```python
from build123d import *

# Parameters (mm, degrees)
SKETCH1_W           = 288.2
SKETCH1_H           = 140
EXTRUDE_5_DEPTH     = 5
SKETCH2_W           = 10
SKETCH2_H           = 60
BOSS_EXTRUDE2_DEPTH = 5
SKETCH3_W           = 27
SKETCH3_H           = 4
SKETCH3_W_2         = 3
SKETCH3_H_2         = 7
CUT_EXTRUDE1_DEPTH  = 5
SKETCH4_R           = 8
CUT_EXTRUDE2_DEPTH  = 5
SKETCH5_R           = 2
CUT_EXTRUDE3_DEPTH  = 5
SKETCH6_W           = 50
SKETCH6_H           = 50
BOSS_EXTRUDE3_DEPTH = 5
LPATTERN1_COUNT     = 2
LPATTERN1_PITCH     = 105
FILLET1_R           = 10
FILLET2_R           = 10


with BuildPart() as part:
    # Sketch1 → Extrude 5 (new body)
    with BuildSketch(Plane(origin=(0, 0, 0), x_dir=(1, 0, 0), z_dir=(0, 1, 0))):
        Rectangle(SKETCH1_W, SKETCH1_H)
    extrude(amount=EXTRUDE_5_DEPTH)

    # Sketch2 → Boss-Extrude2 (add)
    with BuildSketch(Plane(origin=(0, 5, 0), x_dir=(1, 0, 0), z_dir=(0, 1, 0))):
        with Locations((144.1, 0)):
            Rectangle(SKETCH2_W, SKETCH2_H)
    boss_extrude2 = extrude(amount=-BOSS_EXTRUDE2_DEPTH)

    # Mirror1: Boss-Extrude2 across plane
    add(boss_extrude2.mirror(Plane(origin=(0, 0, 0), x_dir=(0, 0, 1), z_dir=(1, 0, 0))))

    # Sketch3 → Cut-Extrude1 (cut)
    with BuildSketch(Plane(origin=(0, 5, 0), x_dir=(1, 0, 0), z_dir=(0, 1, 0))):
        with Locations((144.1, 45)):
            Rectangle(SKETCH3_W, SKETCH3_H)
        with Locations((136.6, 45)):
            Rectangle(SKETCH3_W_2, SKETCH3_H_2)
        with Locations((136.6, -45)):
            Rectangle(SKETCH3_W_2, SKETCH3_H_2)
        with Locations((144.1, -45)):
            Rectangle(SKETCH3_W, SKETCH3_H)
        with Locations((-144.1, -45)):
            Rectangle(SKETCH3_W, SKETCH3_H)
        with Locations((-136.6, -45)):
            Rectangle(SKETCH3_W_2, SKETCH3_H_2)
        with Locations((-136.6, 45)):
            Rectangle(SKETCH3_W_2, SKETCH3_H_2)
        with Locations((-144.1, 45)):
            Rectangle(SKETCH3_W, SKETCH3_H)
    extrude(amount=-CUT_EXTRUDE1_DEPTH, mode=Mode.SUBTRACT)

    # Sketch4 → Cut-Extrude2 (cut)
    with BuildSketch(Plane(origin=(0, 5, 0), x_dir=(1, 0, 0), z_dir=(0, 1, 0))):
        Circle(SKETCH4_R)
    cut_extrude2 = extrude(amount=-CUT_EXTRUDE2_DEPTH, mode=Mode.SUBTRACT)

    # Sketch5 → Cut-Extrude3 (cut)
    with BuildSketch(Plane(origin=(0, 5, 0), x_dir=(1, 0, 0), z_dir=(0, 1, 0))):
        with Locations((-18.25, 0)):
            Circle(SKETCH5_R)
        with Locations((18.25, 0)):
            Circle(SKETCH5_R)
    cut_extrude3 = extrude(amount=-CUT_EXTRUDE3_DEPTH, mode=Mode.SUBTRACT)

    # Sketch6 → Boss-Extrude3 (add)
    with BuildSketch(Plane(origin=(0, 5, 0), x_dir=(1, 0, 0), z_dir=(0, 1, 0))):
        with Locations((-25, 95)):
            Rectangle(SKETCH6_W, SKETCH6_H)
        with Locations((25, 95)):
            Rectangle(SKETCH6_W, SKETCH6_H)
    extrude(amount=-BOSS_EXTRUDE3_DEPTH)

    # LPattern1: Cut-Extrude2, Cut-Extrude3 ×2
    with Locations(*[(0, 0, -i * LPATTERN1_PITCH) for i in range(1, LPATTERN1_COUNT)]):
        add(cut_extrude2, mode=Mode.SUBTRACT)
        add(cut_extrude3, mode=Mode.SUBTRACT)

    # Fillet1
    fillet1_edges = [part.edges().sort_by_distance(p)[0] for p in [
        (-50, 2.5, -70),
        (50, 2.5, -70),
    ]]
    fillet(fillet1_edges, radius=FILLET1_R)

    # Fillet2
    fillet2_edges = [part.edges().sort_by_distance(p)[0] for p in [
        (-50, 2.5, -120),
        (50, 2.5, -120),
    ]]
    fillet(fillet2_edges, radius=FILLET2_R)


solid = part.part
```
Part model, mm, in its own coordinate system. Round coordinates to 2 decimals unless told otherwise and drop trailing zeros. Write each loop counter-clockwise with the first axis right and the second up, starting at its lowest first coordinate (ties: lowest second). Pieces come first, ordered by that corner, then holes. Notation, with made-up numbers: M -3.5,33 L 30.5,33 A31 ccw 30.5,58 Z; hole C 79,-33 d6. An arc over 180 degrees is marked long. One line per question, with ' | ' between items.
(1) Saw through at B-B on y = 3.05. Count the separate pieces of the cut face and the enclosed holes in it, then the cut area to 3 significant figures.
Answer key:
separate pieces: 1 | enclosed holes: 6 | area: 45,200 mm^2
(2) Two-plate mould, pull along X, no slides. Class faces 1 (the face through (-1.73, 2.54, 7.81)), 2 (the face through (2, 5, -26)), 3 (the face through (-53.01, 2.46, -72.85)): released by +X, released by -X, zero draft, split by the parting line, or undercut.
Answer key:
face 1: undercut | face 2: zero draft | face 3: released by -X
(3) Saw through at D-D on z = -77. Write the cut outline in (x, y).
Answer key:
outline: M -50.46,0 L 50.46,0 L 50.46,5 L -50.46,5 Z
(4) Saw through at C-C on x = 93.5. Write the cut outline in (y, z), then the cut area to 3 significant figures.
Answer key:
outline: M 0,-70 L 5,-70 L 5,70 L 0,70 Z | area: 700 mm^2
(5) Probe line 1 along X through (y, z) = (4.25, -42); line 2 along Z through (x, y) = (-18.25, 3.1); line 3 along X through (y, z) = (3.2, -105). List the from-to ranges inside material, lowest first.
Answer key:
line 1: x = -144.1 to -138.1, -135.1 to 135.1, 138.1 to 144.1 | line 2: z = -120 to -107, -103 to -2, 2 to 70 | line 3: x = -50 to -20.25, -16.25 to -8, 8 to 16.25, 20.25 to 50
(6) Pin check, flat tips, straight feed: pin 1 (1.6 mm diameter, centred on y = 2.5, z = 48, fed in from +X); pin 2 (2.5 mm diameter, centred on x = -136, y = 3, fed in from -Z); pin 3 (2.5 mm diameter, centred on x = 147, y = 2, fed in from -Z). Stop position of each tip, or through.
Answer key:
pin 1: stops at x = 144.1 | pin 2: stops at z = -70 | pin 3: stops at z = -30
(7) Saw through at A-A on x = 0. Write the cut outline in (y, z), then the cut area to 3 significant figures.
Answer key:
outline: M 0,-120 L 5,-120 L 5,-113 L 0,-113 Z; M 0,-97 L 5,-97 L 5,-8 L 0,-8 Z; M 0,8 L 5,8 L 5,70 L 0,70 Z | area: 790 mm^2
